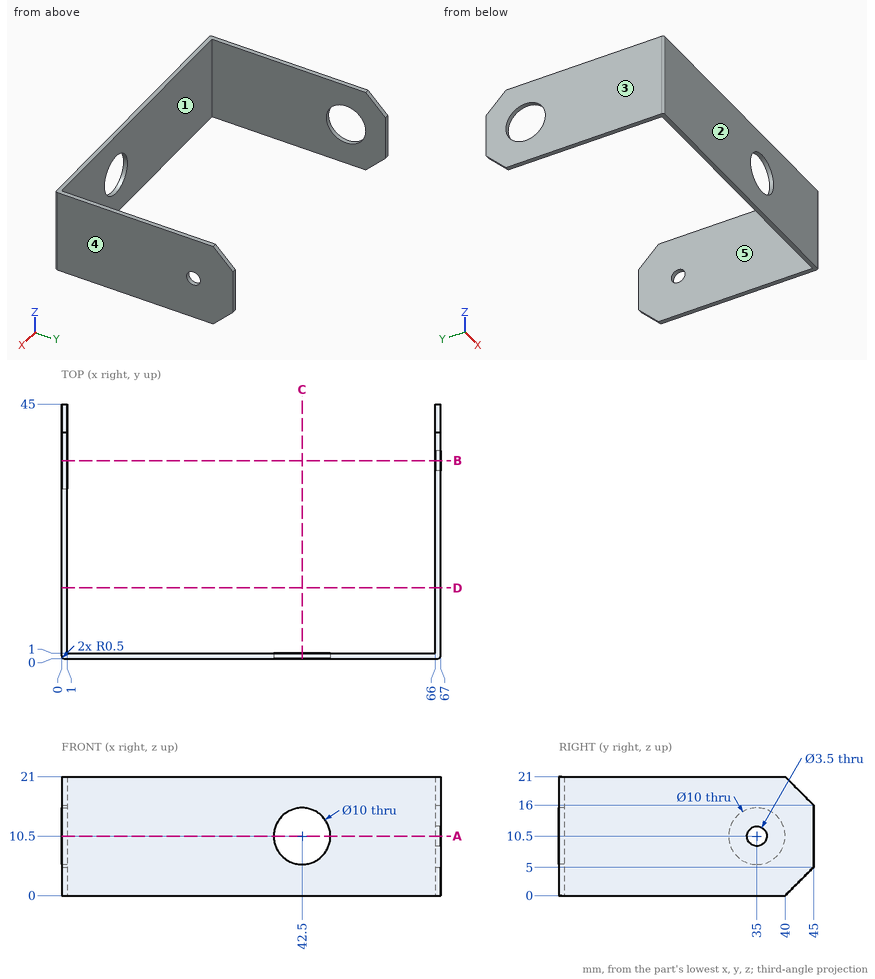
Here's the drawing with two shaded views (mm, measured from the low corner). I have some questions. A direction names the side the tool comes from. Coordinates: 2 decimals unless noted, no trailing zeros. Order: outer loops, then holes, each group sorted by start corner. A loop starts at its lowest first (then second) coordinate and runs counter-clockwise, first axis right, second up. Notation, with made-up numbers: (71.5, 4) -> (124.5, 4) arc R21 cw to (124.5, 18) -> close; hole circle Ø9 at (27.25, 74.5). An arc over 180 degrees is marked (long way). One line per question, with ' | ' between items.
Q1. Thinking about a two-plate mould opening in X: for the marked faces 3, 4 and 5, which applies, pulls with the +X half, pulls with the -X half, needs draft (parallel to the pull), parting line crosses it, or undercut?
Return value:
face 3: pulls with the -X half | face 4: pulls with the +X half | face 5: undercut
Q2. I'm going to push flat-ended pins straight in: P1, Ø3, axis at x = 25.5, z = 15, coming from the +Y side; P2, Ø6, axis at y = 35, z = 10.5, coming from the -X side; P3, Ø12, axis at y = 21.5, z = 16, coming from the -X side. Where does each tip first touch, or does it pass through?
Return value:
P1: y = 1 | P2: x = 66 | P3: x = 0
Q3. Imagine slicing it at B-B on y = 35. Please give me the cut outline in (x, z), and give its area (3 significant figures).
Return value:
outline: (0, 0) -> (1, 0) -> (1, 5.5) -> (0, 5.5) -> close; (0, 15.5) -> (1, 15.5) -> (1, 21) -> (0, 21) -> close; (66, 0) -> (67, 0) -> (67, 8.75) -> (66, 8.75) -> close; (66, 12.25) -> (67, 12.25) -> (67, 21) -> (66, 21) -> close | area: 28.5 mm²
Q4. Imagine slicing it at D-D on y = 12.5. Please give me the cut outline in (x, z).
Return value:
outline: (0, 0) -> (1, 0) -> (1, 21) -> (0, 21) -> close; (66, 0) -> (67, 0) -> (67, 21) -> (66, 21) -> close
Q5. If I drill on L1, parallel to X at y = 8.5, z = 14.25; L2, parallel to Z at x = 42.5, y = 0.45; L3, parallel to X at y = 31, z = 10.5, over which ranges is the centre line in solid material (lowest first)?
Return value:
L1: 0 to 1, 66 to 67 | L2: 0 to 5.5, 15.5 to 21 | L3: 66 to 67
Q6. Imagine slicing it at C-C on x = 42.5. Please give me the cut outline in (y, z), and give its area (3 significant figures).
Return value:
outline: (0, 0) -> (1, 0) -> (1, 5.5) -> (0, 5.5) -> close; (0, 15.5) -> (1, 15.5) -> (1, 21) -> (0, 21) -> close | area: 11.0 mm²
Q7. Imagine slicing it at A-A on z = 10.5. Please give me the cut outline in (x, y), and give its area (3 significant figures).
Return value:
outline: (0, 0.5) arc R0.5 ccw to (0.5, 0) -> (37.5, 0) -> (37.5, 1) -> (1, 1) -> (1, 30) -> (0, 30) -> close; (0, 40) -> (1, 40) -> (1, 45) -> (0, 45) -> close; (47.5, 0) -> (66.5, 0) arc R0.5 ccw to (67, 0.5) -> (67, 33.25) -> (66, 33.25) -> (66, 1) -> (47.5, 1) -> close; (66, 36.75) -> (67, 36.75) -> (67, 45) -> (66, 45) -> close | area: 131 mm²
Q8. On a 3-axis mill with a long thin cutter (end or side, diameter ignored), from which of +Z, -Z, +X, -X, +Y, -Y can I reach the whole of each face in a straight line? I mean the marked faces 1 and 2. Say none if no direction works.
Return value:
face 1: +Z, -Z, +Y | face 2: +Z, -Z, +X, -X, -Y
